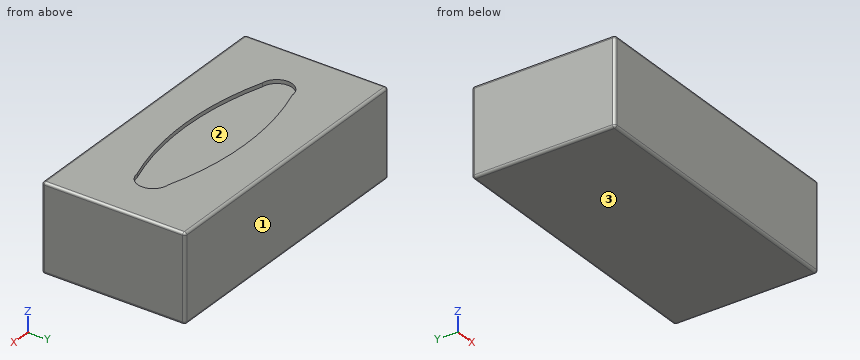
```python
from build123d import *

# Parameters (mm, degrees)
F0_W     = 230
F0_H     = 115
F1_DEPTH = 70
F2_R     = 2
F4_DEPTH = 3


with BuildPart() as f1:
    # F0 (on Top) → F1 (new body)
    with BuildSketch(Plane.XY):
        with Locations((115, 57.5)):
            Rectangle(F0_W, F0_H)
    extrude(amount=F1_DEPTH)

    # F2
    f2_edges = [f1.edges().sort_by_distance(p)[0] for p in [
        (0, 57.5, 70),
        (115, 0, 70),
        (230, 57.5, 70),
        (115, 115, 70),
        (0, 57.5, 0),
        (115, 0, 0),
        (230, 57.5, 0),
        (115, 115, 0),
        (230, 0, 35),
        (230, 115, 35),
        (0, 115, 35),
        (0, 0, 35),
    ]]
    fillet(f2_edges, radius=F2_R)

    # F3 (on face) → F4 (cut)
    with BuildSketch(Plane.XY.offset(70)):
        with BuildLine():
            ThreePointArc((185.3419, 69.995323), (115.162282, 81.286695), (44.981913, 69.999987))
            ThreePointArc((44.981913, 69.999987), (32.520736, 58.219704), (43.545014, 45.084968))
            ThreePointArc((43.545014, 45.084968), (114.480414, 33.514818), (185.42843, 45.007344))
            ThreePointArc((185.42843, 45.007344), (197.499925, 57.543286), (185.3419, 69.995323))
        make_face()
    extrude(amount=-F4_DEPTH, mode=Mode.SUBTRACT)


solid = f1.part
```
Geometry: final body of the model. Coordinates: model frame, mm. Face numbers are marked on the shaded views. Give positions to 0.01 mm unless a question says otherwise; leave off trailing zeros. Loops run counter-clockwise (first coordinate to the right, second up) from the corner with the lowest first, then second, coordinate; pieces in that order, holes last. Notation, with made-up numbers: (43.5, -1.75) -> (77.5, -1.75) arc R23 cw to (77.5, 30.25) -> close; hole circle Ø8 at (41.25, 49). An arc over 180 degrees is marked (long way). Return JSON: item names as keys, results as strings.
Item 1: Pin query (flat end, axial travel): P1, Ø6, axis at x = 148.5, y = 60, coming from the +Z side. Return the tip coordinate at first contact, or that it passes through.
Filled in:
{"P1": "z = 67"}
Item 2: Line query: line 1 (Z direction, x = 134.5, y = 53.5). Output: solid intervals per line, ascending.
Filled in:
{"line 1": "0 to 67"}
Item 3: Section B-B, the plane x = 145. Output: boundary loops of the cut face in (y, z).
Filled in:
{"outline": "(0, 2) arc R2 ccw to (2, 0) -> (113, 0) arc R2 ccw to (115, 2) -> (115, 68) arc R2 ccw to (113, 70) -> (79.29, 70) -> (79.29, 67) -> (35.59, 67) -> (35.59, 70) -> (2, 70) arc R2 ccw to (0, 68) -> close"}
Item 4: Mould query, pull axis Y, two halves, no side actions, for the marked faces 1, 2 and 3. Classes: released by +Y, released by -Y, zero draft, split by the parting line, or undercut.
Filled in:
{"face 1": "released by +Y", "face 2": "undercut", "face 3": "zero draft"}
Item 5: Section A-A, the plane y = 57.5. Output: boundary loops of the cut face in (x, z).
Filled in:
{"outline": "(0, 2) arc R2 ccw to (2, 0) -> (228, 0) arc R2 ccw to (230, 2) -> (230, 68) arc R2 ccw to (228, 70) -> (197.5, 70) -> (197.5, 67) -> (32.5, 67) -> (32.5, 70) -> (2, 70) arc R2 ccw to (0, 68) -> close"}
